Geometry check sheet. Reference: the model listing, model coordinates, mm. Coordinates: 2 decimals unless noted, no trailing zeros. Write each loop counter-clockwise with the first axis right and the second up, starting at its lowest first coordinate (ties: lowest second). Pieces come first, ordered by that corner, then holes. Notation, with made-up numbers: M 70.5,16.25 L 113.5,16.25 A16 ccw 113.5,25.25 Z; hole C 60,89.25 d11. An arc over 180 degrees is marked long. Write item = value, one per line. Start each with the question number.
```python
from build123d import *

# Parameters (mm, degrees)
F0_W        = 92.8924418986
F0_H        = 95.79378739
F1_DEPTH    = 98.552
F2_DEPTH    = 86.106
F3_R        = 12.3937050542
F4_DEPTH    = 203.2
F5_R        = 12.4518339151
F6_DEPTH    = 203.2
F7_T1_DEPTH = 546.6680230822
F8_T1_DEPTH = 558.9322279791


# Not quite as in the source:
# - a fillet or chamfer that OpenCascade refuses, or shapes differently, is made with other operations: its cross-section is extruded or revolved along the edge and cut away or added


with BuildPart() as f1:
    # F0 (on Front) → F1 (new body)
    with BuildSketch(Plane.XZ):
        with Locations((-6.0582030565, -12.6477908343)):
            Rectangle(F0_W, F0_H)
    extrude(amount=F1_DEPTH)

    # F2 (add): a face of the model
    f2_faces = [f1.faces().sort_by_distance(p)[0] for p in [
        (-6.0582030565, 0, -12.6477908343),
    ]]
    extrude(f2_faces, amount=F2_DEPTH)

    # F3 (on face) → F4 (cut)
    with BuildSketch(Plane.XZ.offset(98.552)):
        with Locations((-14.8652456701, -2.7690164279)):
            Circle(F3_R)
    extrude(amount=-F4_DEPTH, mode=Mode.SUBTRACT)

    # F5 (on face) → F6 (cut)
    with BuildSketch(Plane.XZ.offset(98.552)):
        with Locations((3.47437663, -22.2978685051)):
            Circle(F5_R)
    extrude(amount=-F6_DEPTH, mode=Mode.SUBTRACT)

    # F7: fillet of radius 90.7551162367 on 1 edges, made by hand

    # F7_s2 → F7_t1 (cut)
    with BuildSketch(Plane.YZ.offset(-279.3922145976)):
        with BuildLine():
            ThreePointArc((-7.7968837633, 35.2491028607), (-71.9704418816, 8.6675447423), (-98.552, -55.506013376))
            Line((-98.552, -55.506013376), (-98.552, 35.2491028607))
            Line((-98.552, 35.2491028607), (-7.7968837633, 35.2491028607))
        make_face()
    extrude(amount=F7_T1_DEPTH, mode=Mode.SUBTRACT)

    # F8: fillet of radius 93.2079572161 on 1 edges, made by hand

    # F8_s2 → F8_t1 (cut)
    with BuildSketch(Plane.YZ.offset(-285.524317046)):
        with BuildLine():
            ThreePointArc((-7.1019572161, 35.2491028607), (58.8060213919, 7.9491242526), (86.106, -57.9588543554))
            Line((86.106, -57.9588543554), (86.106, 35.2491028607))
            Line((86.106, 35.2491028607), (-7.1019572161, 35.2491028607))
        make_face()
    extrude(amount=F8_T1_DEPTH, mode=Mode.SUBTRACT)


solid = f1.part
```
Q1. Gauge pin test, flat ends, axial feed: pin 1 (10 mm diameter, centred on x = 9, z = -8.5, fed in from +Y); pin 2 (3 mm diameter, centred on x = -34.5, z = -17.5, fed in from -Y); pin 3 (8 mm diameter, centred on x = -25.5, z = -19.5, fed in from +Y). Record the tip position at first contact, or that the pin passes through.
Q2. Cross-section at D-D on z = -29. Enter the section's corners in (x, y).
Q3. Cross-section at B-B on x = -14.5. Enter the section's corners in (y, z).
Q4. Draft check along Z on faces 1 (the face through (-17.55, -7.85, -14.87)), 2 (the face through (-7, -8, -60.545)), 3 (the face through (-6.71, 58.08, 8.67)). Enter one of: pulls with the +Z half, pulls with the -Z half, needs draft (parallel to the pull), parting line crosses it, or undercut.
Q5. Cross-section at A-A on z = -12. Enter the section's corners in (x, y).
Q6. Cross-section at C-C on y = -44.5. Enter the section's corners in (x, z), and give its area (3 significant figures).
Q7. Scan lines: L1, parallel to Z at x = -7, y = 19; L2, parallel to Z at x = 7, y = 18; L3, parallel to Z at x = -23.5, y = -73. Record each from-to range of solid material in increasing order.
Values found:
q1.pin_1 = 74.44
q1.pin_2 = -90.89
q1.pin_3 = 79.5
q2.outline = M -52.5,-94.6 L -7.02,-94.6 L -7.02,81.49 L -52.5,81.49 Z; M 13.97,-94.6 L 40.39,-94.6 L 40.39,81.49 L 13.97,81.49 Z
q3.outline = M -98.55,-60.54 L 86.11,-60.54 L 86.11,-57.96 A93.21 ccw 75.7,-15.16 L -89.09,-15.16 A90.76 ccw -98.55,-55.51 Z; M -71,9.62 L 57.09,9.62 A93.21 ccw -7.1,35.25 L -7.8,35.25 A90.76 ccw Z
q4.face_1 = undercut
q4.face_2 = pulls with the -Z half
q4.face_3 = pulls with the +Z half
q5.outline = M -52.5,-87.44 L -23.14,-87.44 L -23.14,73.99 L -52.5,73.99 Z; M -6.6,-87.44 L -3.53,-87.44 L -3.53,73.99 L -6.6,73.99 Z; M 10.47,-87.44 L 40.39,-87.44 L 40.39,73.99 L 10.47,73.99 Z
q6.outline = M -52.5,-60.54 L 40.39,-60.54 L 40.39,27.5 L -52.5,27.5 Z; hole C -14.87,-2.77 d24.79; hole C 3.47,-22.3 d24.9
q6.area = 7,210 mm²
q7.L1 = -60.54 to -29.03, -15.56 to -12.35, 6.81 to 31.52
q7.L2 = -60.54 to -34.24, -10.36 to 31.81
q7.L3 = -60.54 to -11.66, 6.12 to 7.62
